Part print with two shaded views. Sizes in mm from the minimum x, y, z corner. Give positions to 0.01 mm unless a question says otherwise; leave off trailing zeros. Write each loop counter-clockwise with the first axis right and the second up, starting at its lowest first coordinate (ties: lowest second). Pieces come first, ordered by that corner, then holes. Notation, with made-up numbers: (68.5, 58.25) - (79.5, 58.25) arc R13 cw to (79.5, 72.25) - close; hole circle Ø2 at (68.25, -24.5). An arc over 180 degrees is marked (long way). One line per item, written item: value. Start each with the question number.
(1) Probe L1, parallel to X at y = 5, z = 161.5; L2, parallel to X at y = 3, z = 148.5; L3, parallel to Z at x = 292, y = 5.5. List the from-to ranges inside material, lowest first.
(2) Drop flat-ended pins along their axis: P1, Ø3, axis at x = 269.5, y = 3, coming from the -Z side; P2, Ø3, axis at y = 4, z = 225.5, coming from the -X side; P3, Ø1.5, axis at y = 4, z = 215, coming from the -X side. Give the stop position or say it passes through.
(3) Cut at B-B, the plane x = 58. List the corners of the cut face in (y, z).
(4) Cut at D-D, the plane z = 277.5. List the corners of the cut face in (x, y).
(5) Cut at A-A, the plane z = 177.8. List the corners of the cut face in (x, y), and give its area (3 significant figures).
(6) Cut at C-C, the plane y = 5. State how many separate pieces and enclosed holes the cut face has, and give its area (3 significant figures).
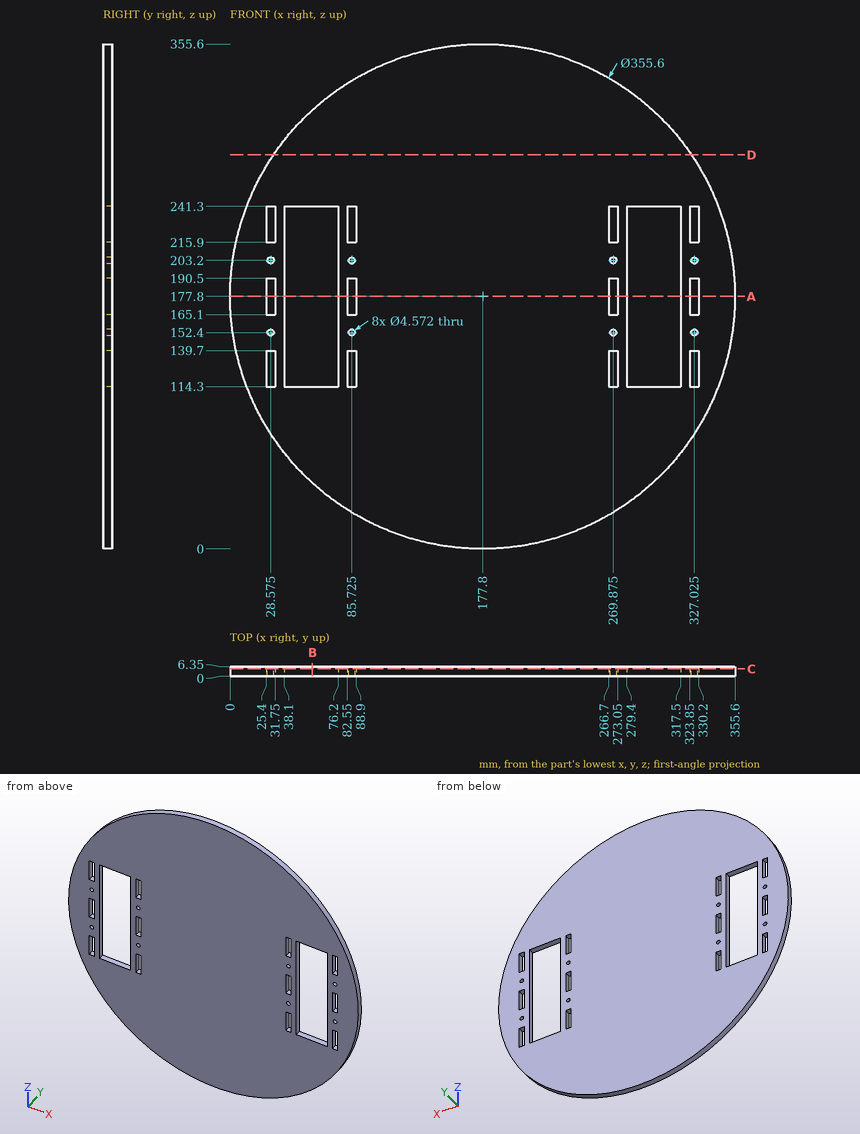
Answers follow:
1. L1: x = 0.75 to 38.1, 76.2 to 279.4, 317.5 to 354.85
1. L2: x = 2.43 to 38.1, 76.2 to 279.4, 317.5 to 353.17
1. L3: z = 41.52 to 114.3, 241.3 to 314.08
2. P1: stops at z = 24.58
2. P2: stops at x = 6.11
2. P3: stops at x = 3.78
3. outline: (0, 46.42) - (6.35, 46.42) - (6.35, 114.3) - (0, 114.3) - close; (0, 241.3) - (6.35, 241.3) - (6.35, 309.18) - (0, 309.18) - close
4. outline: (30.58, 0) - (325.02, 0) - (325.02, 6.35) - (30.58, 6.35) - close
5. outline: (0, 0) - (25.4, 0) - (25.4, 6.35) - (0, 6.35) - close; (31.75, 0) - (38.1, 0) - (38.1, 6.35) - (31.75, 6.35) - close; (76.2, 0) - (82.55, 0) - (82.55, 6.35) - (76.2, 6.35) - close; (88.9, 0) - (266.7, 0) - (266.7, 6.35) - (88.9, 6.35) - close; (273.05, 0) - (279.4, 0) - (279.4, 6.35) - (273.05, 6.35) - close; (317.5, 0) - (323.85, 0) - (323.85, 6.35) - (317.5, 6.35) - close; (330.2, 0) - (355.6, 0) - (355.6, 6.35) - (330.2, 6.35) - close
5. area: 1,610 mm²
6. separate pieces: 1
6. enclosed holes: 22
6. area: 87,600 mm²
